from build123d import *

# Parameters (mm, degrees)
SKETCH_1_W        = 30
SKETCH_1_H        = 120
EXTRUDE_1_DEPTH   = 1.05
EXTRUDE_1_2_DEPTH = 2.1
EXTRUDE_START     = -2.1
EXTRUDE_3_DEPTH   = 2.1
FILLET_1_R        = 1
FILLET_2_R        = 2
FILLET_3_R        = 1


# Read off the part's stored shape, not the designer's step: 拉伸-薄壁3
with BuildPart() as part:
    # 草图1 → Extrude 1 (new, symmetric)
    with BuildSketch(Plane.XY):
        with BuildLine():
            Line((20, -68), (20, 67))
            Line((20, 67), (10, 67))
            Line((10, 67), (10, 65.707106781))
            ThreePointArc((10, 65.707106781), (10, 65), (9.292893219, 65))
            Line((9.292893219, 65), (-9.292893219, 65))
            ThreePointArc((-9.292893219, 65), (-10, 65), (-10, 65.707106781))
            Line((-10, 65.707106781), (-10, 67))
            Line((-10, 67), (-20, 67))
            Line((-20, 67), (-20, -68))
            Line((-20, -68), (-10, -68))
            Line((-10, -68), (-10, -65.707106781))
            ThreePointArc((-10, -65.707106781), (-10, -65), (-9.292893219, -65))
            Line((-9.292893219, -65), (9.292893219, -65))
            ThreePointArc((9.292893219, -65), (10, -65), (10, -65.707106781))
            Line((10, -65.707106781), (10, -68))
            Line((10, -68), (20, -68))
        make_face()
        Rectangle(SKETCH_1_W, SKETCH_1_H, mode=Mode.SUBTRACT)
    extrude(amount=EXTRUDE_1_DEPTH, both=True)

    # 草图2 → Extrude 1 2 (add)
    with BuildSketch(Plane.XY.offset(1.05)):
        Polygon((13.54478625, 60.363803438), (-16.45521375, -59.636196562), (-13.54478625, -60.363803438), (16.45521375, 59.636196562), align=None)
        Polygon((16.45521375, -59.636196562), (-13.54478625, 60.363803438), (-16.45521375, 59.636196562), (13.54478625, -60.363803438), align=None)
    extrude(amount=-EXTRUDE_1_2_DEPTH)

    # 拉伸-薄壁3 outline → 拉伸-薄壁3 (add)
    with BuildSketch(Plane.XY.offset(1.05).offset(EXTRUDE_START)):
        Polygon((15, 1), (1.79616461, 1), (1.54616461, 0), (1.79616461, -1), (15, -1), align=None)
        Polygon((-1.79616461, 1), (-15, 1), (-15, -1), (-1.79616461, -1), (-1.54616461, 0), align=None)
        Polygon((1, 46.191241385), (1, 60), (-1, 60), (-1, 46.191241385), (-7.281623132, 35.311150966), (-6.583792611, 32.519828883), (0, 43.923292192), (6.583792611, 32.519828883), (7.281623132, 35.311150966), align=None)
    extrude_3 = extrude(amount=EXTRUDE_3_DEPTH)

    # 镜向1: 拉伸-薄壁3 across plane
    add(extrude_3.mirror(Plane.ZX))

    # 圆角1
    fillet_1_edges = [part.edges().sort_by_distance(p)[0] for p in [
        (15, 53.815341562, 0),
        (0, 6.184658438, 0),
        (15, -53.815341562, 0),
        (0, -6.184658438, 0),
        (-15, -53.815341562, 0),
        (-15, 53.815341562, 0),
    ]]
    fillet(fillet_1_edges, radius=FILLET_1_R)

    # 圆角2
    fillet_2_edges = [part.edges().sort_by_distance(p)[0] for p in [
        (13.45383539, -60, 0),
        (-13.45383539, -60, 0),
        (-13.45383539, 60, 0),
        (13.45383539, 60, 0),
        (1.79616461, 1, 0),
        (1.79616461, -1, 0),
        (-1.79616461, -1, 0),
        (-1.79616461, 1, 0),
        (-15, 1, 0),
        (15, 1, 0),
        (-15, -1, 0),
        (15, -1, 0),
        (6.583792611, 32.519828883, 0),
        (-6.583792611, 32.519828883, 0),
        (1, 60, 0),
        (-1, 60, 0),
        (-1, 46.191241385, 0),
        (1, 46.191241385, 0),
        (-6.583792611, -32.519828883, 0),
        (6.583792611, -32.519828883, 0),
        (1, -46.191241385, 0),
        (-1, -46.191241385, 0),
        (-1, -60, 0),
        (1, -60, 0),
    ]]
    fillet(fillet_2_edges, radius=FILLET_2_R)

    # 圆角3
    fillet_3_edges = [part.edges().sort_by_distance(p)[0] for p in [
        (7.281623132, 35.311150966, 0),
        (-7.281623132, 35.311150966, 0),
        (0, 43.923292192, 0),
        (-7.281623132, -35.311150966, 0),
        (7.281623132, -35.311150966, 0),
        (0, -43.923292192, 0),
    ]]
    fillet(fillet_3_edges, radius=FILLET_3_R)


solid = part.part
Work out the finished part from the listing and answer in its coordinate system (mm). A direction names the side the tool comes from. Coordinates: 2 decimals unless noted, no trailing zeros. Write each loop counter-clockwise with the first axis right and the second up, starting at its lowest first coordinate (ties: lowest second). Pieces come first, ordered by that corner, then holes.
1. For faces 1 (the flat face through (-3.64, 20.75, 0.01)), 2 (the flat face through (0, 0, 1.05)), determine the directions among +Z, -Z, +X, -X, +Y, -Y from which every point of the face is accessible in a straight line to the end or side of a thin tool.
Results list:
face 1: +Z, -Z
face 2: +Z, +X, -X, +Y, -Y
2. For a pull along X with two mould halves and no side action, classify faces 3 (the flat face through (0, 0, -1.05)), 4 (the flat face through (10.32, -47.47, 0.01)) as +X half, -X half, draft (parallel to the pull), parting line (faces both ways), or undercut.
Results list:
face 3: draft
face 4: undercut
3. Consider line 1 along Y through (x, z) = (-14, -0.45); line 2 along X through (y, z) = (-55.5, 0.05); line 3 along X through (y, z) = (-16, 0.75). Determine where each line is inside the solid, lowest interval first.
Results list:
line 1: y = -68 to -46.69, -1.27 to 1.27, 46.69 to 67
line 2: x = -20 to -12.33, -1 to 1, 12.33 to 20
line 3: x = -20 to -15, -5.55 to -2.45, 2.45 to 5.55, 15 to 20
4. The part is cut by section B-B, the plane z = -0.5. State how many separate pieces and enclosed holes the cut face has, and give its area (3 significant figures).
Results list:
separate pieces: 1
enclosed holes: 10
area: 2,680 mm2
5. The part is cut by section A-A, the plane y = -19.5. Write down the section's boundary in (x, z).
Results list:
outline: (-20, -1.05) - (-15, -1.05) - (-15, 1.05) - (-20, 1.05) - close; (-6.42, -1.05) - (-3.33, -1.05) - (-3.33, 1.05) - (-6.42, 1.05) - close; (3.33, -1.05) - (6.42, -1.05) - (6.42, 1.05) - (3.33, 1.05) - close; (15, -1.05) - (20, -1.05) - (20, 1.05) - (15, 1.05) - close
6. Flat-ended cylindrical pins translate along their axes: pin 1 (1 mm diameter, centred on x = 4, z = 0.5, fed in from -Y); pin 2 (1 mm diameter, centred on x = 8.5, z = 0.5, fed in from +Y). Find the tip coordinate at first contact, or state that the pin passes through.
Results list:
pin 1: stops at y = -65
pin 2: stops at y = 65
